Build history of the part. All positions in model axes, mm. A direction names the side the tool comes from. Give positions to 0.01 mm unless a question says otherwise; leave off trailing zeros. Write each loop counter-clockwise with the first axis right and the second up, starting at its lowest first coordinate (ties: lowest second). Pieces come first, ordered by that corner, then holes. Notation, with made-up numbers: (54.25, 30) -> (100.25, 30) arc R20 ccw to (100.25, 61) -> close; hole circle Ø11 at (79, 63). An arc over 180 degrees is marked (long way). One line per question, with ' | ' between items. Start each with the question number.
(1) Pull direction X, two halves, no side cores. Call faces 4 (the cylindrical face through (-3, 0, 12)), 5 (the flat face through (-2.41, 0.24, 1.48)), 6 (the flat face through (2, 2, 0)): released by +X, released by -X, zero draft, split by the parting line, or undercut.
(2) Pin check, flat tips, straight feed: P1, Ø3, axis at y = -1.5, z = 7.5, coming from the -X side; P2, Ø1.5, axis at x = 1, y = -1, coming from the -Z side. Stop position of each tip, or through.
(3) Band-saw the part on C-C, the plane x = -1.5. Give the cut face in (y, z), and give its area (3 significant figures).
(4) Band-saw the part on A-A, the plane z = 2. Give the cut face in (x, y), and give its area (3 significant figures).
(5) Band-saw the part on B-B, the plane y = 2. Give the cut face in (x, z).
(6) Tool access for faces 1 (the flat face through (0, 0, 20)), 2 (the flat face through (1, 3, 5)), 3 (the flat face through (-1.41, -1.97, 1.48)): list every direction of +Z, -Z, +X, -X, +Y, -Y with a clear straight run to the whole face (end or side of a thin tool).
(7) Band-saw the part on D-D, the plane z = 19.25. Give the cut face in (x, y), and give its area (3 significant figures).
(8) Drill centre lines: probe 1 along Z at (x, y) = (1.25, 0); probe 2 along X at (y, z) = (1.25, 2.25); probe 3 along Z at (x, y) = (1.75, 2.5). Where is each one in solid material? Low to high. Write a range as from..to.
from build123d import *

# Parameters (mm, degrees)
SKETCH1_R           = 4
BOSS_EXTRUDE1_DEPTH = 5
SKETCH2_R           = 3
BOSS_EXTRUDE2_DEPTH = 15
CUT_EXTRUDE1_DEPTH  = 3


with BuildPart() as part:
    # Sketch1 → Boss-Extrude1 (new body)
    with BuildSketch(Plane.XY):
        Circle(SKETCH1_R)
    extrude(amount=BOSS_EXTRUDE1_DEPTH)

    # Sketch2 → Boss-Extrude2 (add)
    with BuildSketch(Plane.XY.offset(5)):
        Circle(SKETCH2_R)
    extrude(amount=BOSS_EXTRUDE2_DEPTH)

    # Sketch3 → Cut-Extrude1 (cut)
    with BuildSketch(Plane(origin=(0, 0, 0), x_dir=(-1, 0, 0), z_dir=(0, 0, -1))):
        Polygon((0.294791558, -2.782244545), (2.556890234, -1.135825295), (2.262098677, 1.64641925), (-0.294791558, 2.782244545), (-2.556890234, 1.135825295), (-2.262098677, -1.64641925), align=None)
    extrude(amount=-CUT_EXTRUDE1_DEPTH, mode=Mode.SUBTRACT)


solid = part.part
Results:
1) face 4: split by the parting line | face 5: undercut | face 6: zero draft
2) P1: stops at x = -3 | P2: stops at z = 3
3) outline: (-3.71, 0) -> (-1.91, 0) -> (-1.91, 3) -> (1.98, 3) -> (1.98, 0) -> (3.71, 0) -> (3.71, 5) -> (2.6, 5) -> (2.6, 20) -> (-2.6, 20) -> (-2.6, 5) -> (-3.71, 5) -> close | area: 103 mm²
4) outline: circle Ø8 at (0, 0); hole (-2.56, -1.14) -> (-0.29, -2.78) -> (2.26, -1.65) -> (2.56, 1.14) -> (0.29, 2.78) -> (-2.26, 1.65) -> close | area: 29.9 mm²
5) outline: (-3.46, 0) -> (-1.47, 0) -> (-1.47, 3) -> (1.37, 3) -> (1.37, 0) -> (3.46, 0) -> (3.46, 5) -> (2.24, 5) -> (2.24, 20) -> (-2.24, 20) -> (-2.24, 5) -> (-3.46, 5) -> close
6) face 1: +Z, +X, -X, +Y, -Y | face 2: +Z | face 3: -Z
7) outline: circle Ø6 at (0, 0) | area: 28.3 mm²
8) probe 1: z = 3..20 | probe 2: x = -3.8..-2.3, 2.4..3.8 | probe 3: z = 0..5
